Input: part model. Units: mm. Frame: model coordinates. Face numbers are marked on the shaded views. Round coordinates to 2 decimals unless told otherwise and drop trailing zeros. Order: outer loops, then holes, each group sorted by start corner. A loop starts at its lowest first (then second) coordinate and runs counter-clockwise, first axis right, second up. Notation, with made-up numbers: (33.25, 23) -> (53.25, 23) arc R10 cw to (53.25, 40) -> close; hole circle Ø9 at (67.5, 85.25). An arc over 180 degrees is marked (long way). Use a Markdown table: item, result.
from build123d import *

# Parameters (mm, degrees)
F0_W     = 55
F0_H     = 18
F0_R     = 1.25
F0_R_2   = 4.4
F0_R_3   = 1.2
F1_DEPTH = 12


with BuildPart() as f1:
    # F0 (on Top) → F1 (new body)
    with BuildSketch(Plane.XY):
        Rectangle(F0_W, F0_H)
        with Locations((-20.5, -6)):
            Circle(F0_R, mode=Mode.SUBTRACT)
        with Locations((17, -1.5)):
            Circle(F0_R_2, mode=Mode.SUBTRACT)
        with Locations((-24.5, 0)):
            Circle(F0_R_3, mode=Mode.SUBTRACT)
        with Locations((-17, 1.5)):
            Circle(F0_R_2, mode=Mode.SUBTRACT)
        Circle(F0_R_2, mode=Mode.SUBTRACT)
        with Locations((20.5, 6)):
            Circle(F0_R, mode=Mode.SUBTRACT)
    extrude(amount=F1_DEPTH)


solid = f1.part
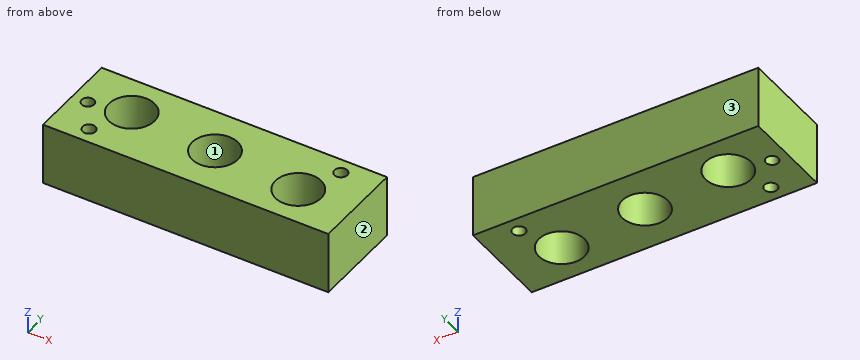
1) Draft query along Y for the marked faces 1, 2 and 3. Return one class per face: released by +Y, released by -Y, zero draft, split by the parting line, or undercut.
Answer key:
| item | result |
|---|---|
| face 1 | undercut |
| face 2 | zero draft |
| face 3 | released by +Y |
2) Cut plane B-B on z = 8.75. Return loops of the section in (x, y), and give its area (3 significant figures).
Answer key:
| item | result |
|---|---|
| outline | (-27.5, -9) -> (27.5, -9) -> (27.5, 9) -> (-27.5, 9) -> close; hole circle Ø2.4 at (-24.5, 0); hole circle Ø2.5 at (-20.5, -6); hole circle Ø8.8 at (-17, 1.5); hole circle Ø8.8 at (0, 0); hole circle Ø8.8 at (17, -1.5); hole circle Ø2.5 at (20.5, 6) |
| area | 793 mm^2 |
3) Cut plane C-C on x = -24.5. Return loops of the section in (y, z).
Answer key:
| item | result |
|---|---|
| outline | (-9, 0) -> (-1.2, 0) -> (-1.2, 12) -> (-9, 12) -> close; (1.2, 0) -> (9, 0) -> (9, 12) -> (1.2, 12) -> close |
4) Ray query, probe 1 along X at (y, z) = (-3.25, 7.5); probe 2 along Y at (x, z) = (0, 5.75); probe 3 along X at (y, z) = (-2, 10.5). Return the intervals inside material, ascending.
Answer key:
| item | result |
|---|---|
| probe 1 | x = -27.5 to -2.97, 2.97 to 12.96, 21.04 to 27.5 |
| probe 2 | y = -9 to -4.4, 4.4 to 9 |
| probe 3 | x = -27.5 to -19.67, -14.33 to -3.92, 3.92 to 12.63, 21.37 to 27.5 |
5) Contact query for flat-ended pins moving along their axis: P1, Ø10, axis at x = 17, y = -1.5, coming from the +Z side; P2, Ø8, axis at x = 0, y = 0, coming from the -Z side. Output: stop coordinate, or through.
Answer key:
| item | result |
|---|---|
| P1 | stops at z = 12 |
| P2 | passes through |
6) Cut plane A-A on x = -17. Return loops of the section in (y, z).
Answer key:
| item | result |
|---|---|
| outline | (-9, 0) -> (-2.9, 0) -> (-2.9, 12) -> (-9, 12) -> close; (5.9, 0) -> (9, 0) -> (9, 12) -> (5.9, 12) -> close |
